Can you work these out from the model? Positions are in its coordinate system, mm. Face numbers are marked on the shaded views. Coordinates: 2 decimals unless noted, no trailing zeros. Order: outer loops, then holes, each group sorted by start corner. A loop starts at its lowest first (then second) coordinate and runs counter-clockwise, first axis right, second up. Notation, with made-up numbers: (-12, 76.5) -> (31, 76.5) arc R21 cw to (31, 83.5) -> close; hole circle Ø2 at (-18, -16). An arc over 180 degrees is marked (long way). Return JSON: item names as keys, results as strings. Group by question number.
1) If we section it at B-B, the plane y = 9.75: Please give me the cut outline in (x, z).
2) For pin 1 (1 mm diameter, centred on y = -3.5, z = 1, fed in from -X); pin 2 (4 mm diameter, centred on x = 3.5, y = -5, fed in from +Z); pin 3 (13.5 mm diameter, centred on x = 32, y = 6, fed in from +Z), each with a flat end and sliding along its axis, tell me the tip position at first contact or that it passes through.
3) If we section it at A-A, the plane x = 40.5: Please give me the cut outline in (y, z).
4) If I drill on probe 1 along Z at (x, y) = (6.5, 5.25); probe 2 along X at (y, z) = (5.75, 8.75); probe 3 along X at (y, z) = (1.25, 19), over which ranges is the centre line in solid material (lowest first)? Write a range as from..to.
5) Thinking about a two-plate mould opening in Y: for the marked faces 1 and 2, which applies, +Y half, -Y half, draft (parallel to the pull), parting line (faces both ways), or undercut?
from build123d import *

# Parameters (mm, degrees)
F1_DEPTH      = 2.4
F4_DEPTH      = 25
F4_DEPTH_BACK = 1
F5_R          = 5
F6_T1_DEPTH   = 77.4
F7_R          = 1
F8_R          = 1.99999
F10_START     = 3
F10_DEPTH     = 22


# Not quite as in the source:
# - a fillet or chamfer that OpenCascade refuses, or shapes differently, is made with other operations: its cross-section is extruded or revolved along the edge and cut away or added
# - a fillet or chamfer is up to 0.001 mm smaller than in the source, because OpenCascade refuses the exact size


with BuildPart() as f1:
    # F0 (on Top) → F1 (new body)
    with BuildSketch(Plane.XY):
        Polygon((70, 13.5), (-10, 13.5), (-10, -13.5), (70, -13.5), (70, -6.5), (50, -6.5), (50, 6.5), (70, 6.5), align=None)
        with BuildLine():
            ThreePointArc((4.75, 0), (0, -4.75), (-4.75, 0))
            Line((-4.75, 0), (0, 6.45))
            Line((0, 6.45), (4.75, 0))
        make_face(mode=Mode.SUBTRACT)
        with BuildLine():
            Line((0, 6.45), (-4.75, 0))
            ThreePointArc((-4.75, 0), (0, -4.75), (4.75, 0))
            Line((4.75, 0), (0, 6.45))
        make_face()
    extrude(amount=-F1_DEPTH)

    # F3 (on line) → F4 (join, two sides)
    with BuildSketch(Plane(origin=(0, 0, 0), x_dir=(0.984807753, 0, -0.1736481777), z_dir=(-0.1736481777, 0, -0.984807753))) as f4_sk:
        with BuildLine():
            ThreePointArc((4.75, 0), (0, 4.75), (-4.75, 0))
            Line((-4.75, 0), (0, -6.45))
            Line((0, -6.45), (4.75, 0))
        make_face()
    extrude(amount=-F4_DEPTH)
    extrude(f4_sk.sketch, amount=F4_DEPTH_BACK)

    # F5
    f5_edges = [f1.edges().sort_by_distance(p)[0] for p in [
        (70, -13.5, -1.2),
        (70, 13.5, -1.2),
    ]]
    fillet(f5_edges, radius=F5_R)

    # F6: fillet of radius 15 on 2 edges, made by hand

    # F6_s2 → F6_t1 (cut)
    with BuildSketch(Plane.XY.offset(-39.9)):
        with BuildLine():
            ThreePointArc((-10, 1.5), (-5.6066017178, -9.1066017178), (5, -13.5))
            Line((5, -13.5), (-10, -13.5))
            Line((-10, -13.5), (-10, 1.5))
        make_face()
        with BuildLine():
            ThreePointArc((5, 13.5), (-5.6066017178, 9.1066017178), (-10, -1.5))
            Line((-10, -1.5), (-10, 13.5))
            Line((-10, 13.5), (5, 13.5))
        make_face()
    extrude(amount=F6_T1_DEPTH, mode=Mode.SUBTRACT)

    # F7
    f7_edges = [f1.edges().sort_by_distance(p)[0] for p in [
        (0, -4.75, 0),
        (-2.411638, 3.225, 0),
        (2.411638, 3.225, 0),
    ]]
    fillet(f7_edges, radius=F7_R)

    # F8 (radius 2 in the source; OpenCascade refuses exactly that, so slightly less here)
    f8_edges = [f1.edges().sort_by_distance(p)[0] for p in [
        (70, 6.5, -1.2),
        (70, -6.5, -1.2),
    ]]
    fillet(f8_edges, radius=F8_R)

    # F9 (on Front) → F10 (cut)
    with BuildSketch(Plane.XZ.offset(F10_START)):
        with BuildLine():
            ThreePointArc((2.1757445863, 12.3392607162), (4.2168340546, 12.8861689909), (5.1098650304, 14.8012800987))
            ThreePointArc((5.1098650304, 14.8012800987), (4.5249761382, 16.4082491229), (3.0439854746, 17.2632994812))
            Line((3.0439854746, 17.2632994812), (2.1757445863, 12.3392607162))
        make_face()
        with BuildLine():
            Line((2.1757445863, 12.3392607162), (3.0439854746, 17.2632994812))
            ThreePointArc((3.0439854746, 17.2632994812), (0.1478456479, 15.2354005429), (2.1757445863, 12.3392607162))
        make_face()
    extrude(amount=F10_DEPTH, mode=Mode.SUBTRACT)


solid = f1.part
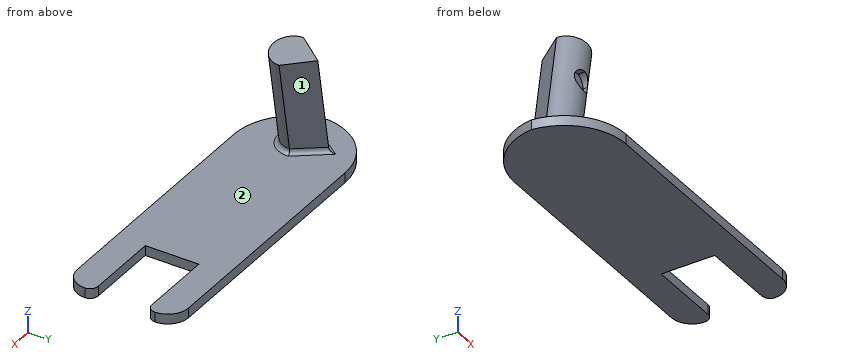
Result sheet:
{
 "1": {"outline": "(-4.92, -2.4) -> (69.84, -2.4) -> (69.84, 0) -> (-4.92, 0) -> close"},
 "2": {"pin 1": "stops at x = -3.57", "pin 2": "stops at z = 25.07", "pin 3": "stops at z = 0"},
 "3": {"outline": "(-13.5, -2.4) -> (13.5, -2.4) -> (13.5, 0) -> (-13.5, 0) -> close"},
 "4": {"probe 1": "z = -2.4..0", "probe 2": "x = 1.02..2.07", "probe 3": "x = -0.54..7.24"},
 "5": {"face 1": "+Y half", "face 2": "draft"}
}
